Input: dimensioned drawing with shaded views. Units: mm. Origin: part minimum x, y, z. Coordinates: 2 decimals unless noted, no trailing zeros. Order: outer loops, then holes, each group sorted by start corner. A loop starts at its lowest first (then second) coordinate and runs counter-clockwise, first axis right, second up. Notation, with made-up numbers: M -39,19 L -3,19 A21 cw -3,30 Z; hole C 24.5,8 d11. An arc over 180 degrees is marked long. Write item = value, one per line.
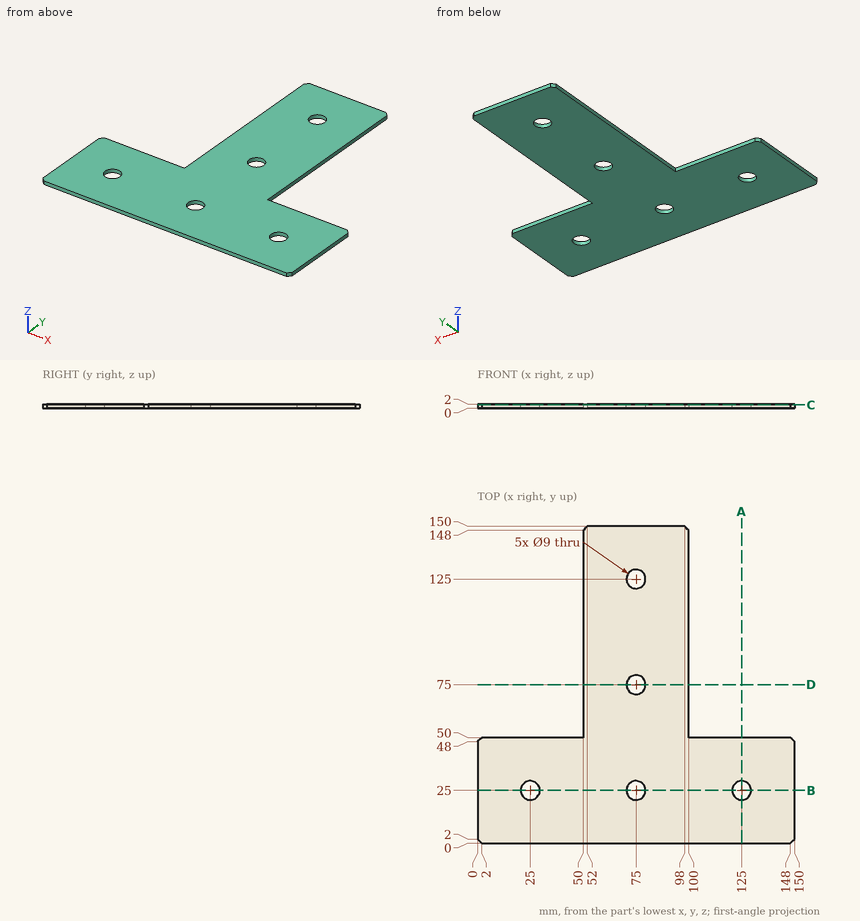
1) Section A-A, the plane x = 125. Return loops of the section in (y, z), and give its area (3 significant figures).
Numbers:
outline = M 0,0 L 20.5,0 L 20.5,2 L 0,2 Z; M 29.5,0 L 50,0 L 50,2 L 29.5,2 Z
area = 82.0 mm²
2) Section B-B, the plane y = 25. Return loops of the section in (x, z).
Numbers:
outline = M 0,0 L 20.5,0 L 20.5,2 L 0,2 Z; M 29.5,0 L 70.5,0 L 70.5,2 L 29.5,2 Z; M 79.5,0 L 120.5,0 L 120.5,2 L 79.5,2 Z; M 129.5,0 L 150,0 L 150,2 L 129.5,2 Z
3) Section C-C, the plane z = 1.55. Return loops of the section in (x, y), and give its area (3 significant figures).
Numbers:
outline = M 0,2 L 2,0 L 148,0 L 150,2 L 150,48 L 148,50 L 100,50 L 100,148 L 98,150 L 52,150 L 50,148 L 50,50 L 2,50 L 0,48 Z; hole C 25,25 d9; hole C 75,25 d9; hole C 75,75 d9; hole C 75,125 d9; hole C 125,25 d9
area = 12,200 mm²
4) Pin query (flat end, axial travel): pin 1 (11.5 mm diameter, centred on x = 75, y = 125, fed in from +Z); pin 2 (1 mm diameter, centred on x = 20.5, z = 1, fed in from +Y); pin 3 (0.6 mm diameter, centred on y = 116, z = 1, fed in from -X). Return the tip coordinate at first contact, or that it passes through.
Numbers:
pin_1 = 2
pin_2 = 50
pin_3 = 50
5) Line query: L1, parallel to Y at x = 75, z = 1.3; L2, parallel to X at y = 75, z = 0.95. Output: solid intervals per line, ascending.
Numbers:
L1 = 0 to 20.5, 29.5 to 70.5, 79.5 to 120.5, 129.5 to 150
L2 = 50 to 70.5, 79.5 to 100
6) Section D-D, the plane y = 75. Return loops of the section in (x, z), and give its area (3 significant figures).
Numbers:
outline = M 50,0 L 70.5,0 L 70.5,2 L 50,2 Z; M 79.5,0 L 100,0 L 100,2 L 79.5,2 Z
area = 82.0 mm²
